```python
from build123d import *

# Parameters (mm, degrees)
BOSS_EXTRUDE2_DEPTH = 0.5
SKETCH3_R           = 1
CUT_EXTRUDE2_DEPTH  = 1.5
FILLET1_R           = 10


with BuildPart() as part:
    # Sketch1 → Boss-Extrude2 (new body)
    with BuildSketch(Plane(origin=(0, 0, 0), x_dir=(1, 0, 0), z_dir=(0, 1, 0))):
        with BuildLine():
            Line((39.801772908, 0), (11.302617333, 4.027174803))
            Line((11.302617333, 4.027174803), (7.464101615, 2))
            Line((7.464101615, 2), (3.464101615, 2))
            ThreePointArc((3.464101615, 2), (-4, 0), (3.464101615, -2))
            Line((3.464101615, -2), (7.464101615, -2))
            Line((7.464101615, -2), (11.302617333, -4.027174803))
            Line((11.302617333, -4.027174803), (39.801772908, 0))
        make_face()
    extrude(amount=BOSS_EXTRUDE2_DEPTH)

    # Sketch3 → Cut-Extrude2 (cut, through all)
    with BuildSketch(Plane(origin=(0, 0.5, 0), x_dir=(1, 0, 0), z_dir=(0, 1, 0))):
        Circle(SKETCH3_R)
    extrude(amount=-CUT_EXTRUDE2_DEPTH, mode=Mode.SUBTRACT)

    # Fillet1
    fillet1_edges = [part.edges().sort_by_distance(p)[0] for p in [
        (3.464101615, 0.25, 2),
        (3.464101615, 0.25, -2),
    ]]
    fillet(fillet1_edges, radius=FILLET1_R)


solid = part.part
```
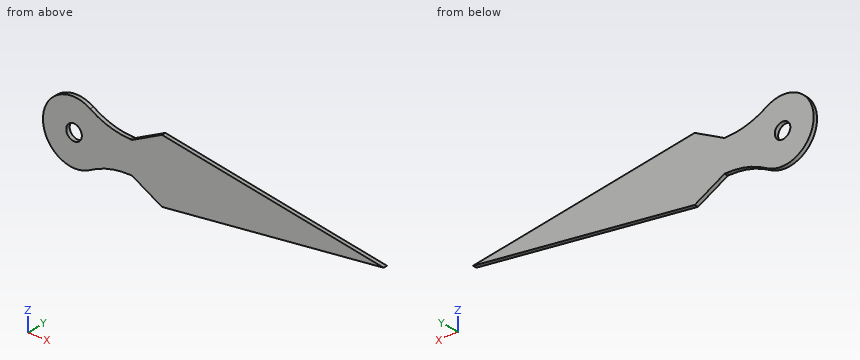
Design review of the part built by this model. Coordinates are the model's own, in mm. Give positions to 0.01 mm unless a question says otherwise; leave off trailing zeros. Order: outer loops, then holes, each group sorted by start corner. A loop starts at its lowest first (then second) coordinate and runs counter-clockwise, first axis right, second up. Notation, with made-up numbers: (82.5, 59.5) -> (137.5, 59.5) arc R30 cw to (137.5, 88.5) -> close; hole circle Ø1 at (50, 88.5). An arc over 180 degrees is marked (long way). Write item = value, one per line. Start each with the question number.
(1) We need section B-B on z = 3. Write out the cut boundary in (x, y), plus the area to 3 significant figures.
(2) We need section A-A on x = 0. Write out the cut boundary in (y, z).
(3) We need section C-C on y = 0.1. Write out the cut boundary in (x, z), plus the area to 3 significant figures.
(4) To check wall thickness, follow line 1 along Z through (x, y) = (0, 0.1); line 2 along Z through (x, y) = (11.5, 0.25); line 3 along Z through (x, y) = (7, 0.1). State the ranges of each line that lie inside material, in increasing order.
(5) We need section D-D on x = 31.5. Write out the cut boundary in (y, z).
Numbers:
q1.outline = (-2.65, 0) -> (2.85, 0) -> (2.85, 0.5) -> (-2.65, 0.5) -> close; (9.36, 0) -> (18.57, 0) -> (18.57, 0.5) -> (9.36, 0.5) -> close
q1.area = 7.36 mm^2
q2.outline = (0, -4) -> (0.5, -4) -> (0.5, -1) -> (0, -1) -> close; (0, 1) -> (0.5, 1) -> (0.5, 4) -> (0, 4) -> close
q3.outline = (2.06, -3.43) arc R10 cw to (7.21, -2) -> (7.46, -2) -> (11.3, -4.03) -> (39.8, 0) -> (11.3, 4.03) -> (7.46, 2) -> (7.21, 2) arc R10 cw to (2.06, 3.43) arc R4 ccw (long way) to start; hole circle Ø2 at (0, 0)
q3.area = 202 mm^2
q4.line_1 = -4 to -1, 1 to 4
q4.line_2 = -4 to 4
q4.line_3 = -2 to 2
q5.outline = (0, -1.17) -> (0.5, -1.17) -> (0.5, 1.17) -> (0, 1.17) -> close
